Read the model definition and answer for the solid it produces. Units are mm, in the model's axes. Coordinates: 2 decimals unless noted, no trailing zeros. Write each loop counter-clockwise with the first axis right and the second up, starting at its lowest first coordinate (ties: lowest second). Pieces come first, ordered by that corner, then holes. Notation, with made-up numbers: (-1, 80) - (39, 80) arc R30 cw to (39, 114) - close; hole circle Ø2 at (-2, -29.5). An arc over 180 degrees is marked (long way). Return JSON: item names as keys, results as strings.
```python
from build123d import *

# Parameters (mm, degrees)
F0_R     = 2.5
F1_DEPTH = 3


with BuildPart() as f1:
    # F0 (on Top) → F1 (new body)
    with BuildSketch(Plane.XY):
        with BuildLine():
            ThreePointArc((-2.5, -40), (0, -37.5), (2.5, -40))
            Line((2.5, -40), (5, -40))
            Line((5, -40), (5, 40))
            Line((5, 40), (-5, 40))
            Line((-5, 40), (-5, -40))
            Line((-5, -40), (-2.5, -40))
        make_face()
        with Locations((0, 35)):
            Circle(F0_R, mode=Mode.SUBTRACT)
        with BuildLine():
            Line((5, -40), (2.5, -40))
            ThreePointArc((2.5, -40), (0, -42.5), (-2.5, -40))
            Line((-2.5, -40), (-5, -40))
            ThreePointArc((-5, -40), (0, -45), (5, -40))
        make_face()
    extrude(amount=F1_DEPTH)


solid = f1.part
```
(1) A cutting plane is placed at B-B (z = 1.25). Determine the outline of the cut face in (x, y), and give its area (3 significant figures).
Answer:
{"outline": "(-5, -40) arc R5 ccw to (5, -40) - (5, 40) - (-5, 40) - close; hole circle Ø5 at (0, -40); hole circle Ø5 at (0, 35)", "area": "800 mm²"}
(2) A cutting plane is placed at A-A (y = 35). Determine the outline of the cut face in (x, z).
Answer:
{"outline": "(-5, 0) - (-2.5, 0) - (-2.5, 3) - (-5, 3) - close; (2.5, 0) - (5, 0) - (5, 3) - (2.5, 3) - close"}
(3) Flat-ended cylindrical pins translate along their axes: P1, Ø6, axis at x = 0, y = -40, coming from the -Z side; P2, Ø4.5, axis at x = 0, y = 35, coming from the -Z side. Find the tip coordinate at first contact, or state that the pin passes through.
Answer:
{"P1": "z = 0", "P2": "through"}
(4) Determine the mould class of faces 1 (the face through (-0.54, 32.56, 1.48)), 2 (the face through (0, -45, 1)), 3 (the face through (5, -1, 1)) for opening direction X: +X half, -X half, draft (parallel to the pull), parting line (faces both ways), or undercut.
Answer:
{"face 1": "undercut", "face 2": "parting line", "face 3": "+X half"}
(5) Straight lines are drawn through the part: line 1 (Y direction, x = 0, z = 0.7); line 2 (X direction, y = -40, z = 1.3); line 3 (Y direction, x = -0.5, z = 0.3). For each, find the intervals that lie inside material, in ascending order. Write a range as from..to.
Answer:
{"line 1": "-45..-42.5, -37.5..32.5, 37.5..40", "line 2": "-5..-2.5, 2.5..5", "line 3": "-44.97..-42.45, -37.55..32.55, 37.45..40"}
(6) A cutting plane is placed at C-C (x = 0). Determine the outline of the cut face in (y, z).
Answer:
{"outline": "(-45, 0) - (-42.5, 0) - (-42.5, 3) - (-45, 3) - close; (-37.5, 0) - (32.5, 0) - (32.5, 3) - (-37.5, 3) - close; (37.5, 0) - (40, 0) - (40, 3) - (37.5, 3) - close"}
(7) A cutting plane is placed at D-D (x = -3.5). Determine the outline of the cut face in (y, z).
Answer:
{"outline": "(-43.57, 0) - (40, 0) - (40, 3) - (-43.57, 3) - close"}
